Geometry check sheet. Reference: the model listing, model coordinates, mm. Face numbers are marked on the shaded views. A direction names the side the tool comes from. Coordinates: 2 decimals unless noted, no trailing zeros. Order: outer loops, then holes, each group sorted by start corner. A loop starts at its lowest first (then second) coordinate and runs counter-clockwise, first axis right, second up. Notation, with made-up numbers: M 76.5,-20.75 L 89.5,-20.75 A8 cw 89.5,-15.75 Z; hole C 58,69.25 d8. An arc over 180 degrees is marked long. One line per item, written item: value. Start each with the question number.
1) Access from +Z, -Z, +X, -X, +Y, -Y to the whole of each face (thin tool, end or side, straight path). Record for the marked faces 1 and 2.
2) Sectioned sample at B-B, the plane x = 0. Enter the section's corners in (y, z).
3) Go/stop test with a flat-tipped pin: P1, Ø9, axis at x = 0, y = 0, coming from the +Z side (3 decimals). Record where the tip stops, or that it passes through.
4) Thickness scan on L1, parallel to Y at x = 0, z = 15; L2, parallel to X at y = 0, z = 1.15; L3, parallel to Y at x = 0, z = 1.35. Record the ranges inside material, lowest first. Write a range as from..to.
5) Sectioned sample at D-D, the plane z = 10.75. Enter the section's corners in (x, y), then the cut area to 3 significant figures.
6) Sectioned sample at C-C, the plane x = 15. Enter the section's corners in (y, z), then the cut area to 3 significant figures.
7) Sectioned sample at A-A, the plane y = -1.75. Enter the section's corners in (x, z), then the cut area to 3 significant figures.
8) Draft check along Y on the marked faces 3, 4, 5 and 6. Enter one of: pulls with the +Y half, pulls with the -Y half, needs draft (parallel to the pull), parting line crosses it, or undercut.
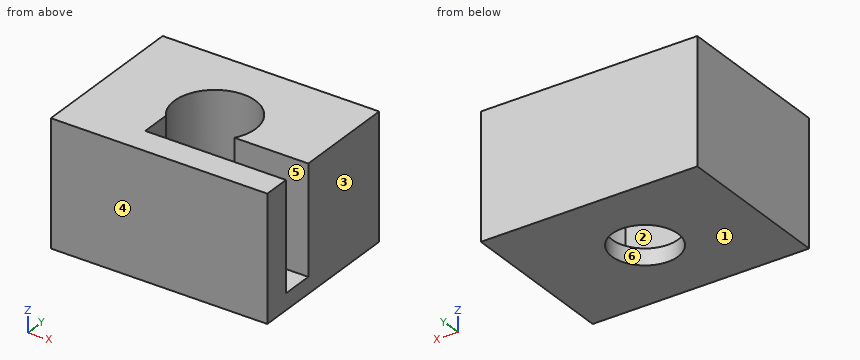
```python
from build123d import *

# Parameters (mm, degrees)
SKETCH1_W           = 40
SKETCH1_H           = 30
BOSS_EXTRUDE1_DEPTH = 23
SKETCH3_R           = 6.1
CUT_EXTRUDE1_DEPTH  = 24
CUT_EXTRUDE2_DEPTH  = 20


with BuildPart() as part:
    # Sketch1 → Boss-Extrude1 (new body)
    with BuildSketch(Plane.XY):
        Rectangle(SKETCH1_W, SKETCH1_H)
    extrude(amount=BOSS_EXTRUDE1_DEPTH)

    # Sketch3 → Cut-Extrude1 (cut, through all)
    with BuildSketch(Plane.XY.offset(23)):
        Circle(SKETCH3_R)
    extrude(amount=-CUT_EXTRUDE1_DEPTH, mode=Mode.SUBTRACT)

    # Sketch4 → Cut-Extrude2 (cut)
    with BuildSketch(Plane.XY.offset(23)):
        with BuildLine():
            Line((-6, -4.5), (-6, -4))
            Line((-6, -4), (-4.605431576, -4))
            ThreePointArc((-4.605431576, -4), (-2.135048874, 5.714154907), (6.1, 0))
            ThreePointArc((6.1, 0), (5.714154907, -2.135048874), (4.605431576, -4))
            Line((4.605431576, -4), (6.34428877, -4))
            ThreePointArc((6.34428877, -4), (7.205281597, -2.081806214), (7.5, 0))
            ThreePointArc((7.5, 0), (-2.371708245, 7.115124735), (-6, -4.5))
        make_face()
        with BuildLine():
            Line((-4.605431576, -4), (-6, -4))
            Line((-6, -4), (-6, -4.5))
            ThreePointArc((-6, -4.5), (0.303535318, -7.493855237), (6.34428877, -4))
            Line((6.34428877, -4), (4.605431576, -4))
            ThreePointArc((4.605431576, -4), (0, -6.1), (-4.605431576, -4))
        make_face()
        with BuildLine():
            ThreePointArc((6.34428877, -4), (0.303535318, -7.493855237), (-6, -4.5))
            Line((-6, -4.5), (-6, -10))
            Line((-6, -10), (20, -10))
            Line((20, -10), (20, -4))
            Line((20, -4), (6.34428877, -4))
        make_face()
    extrude(amount=-CUT_EXTRUDE2_DEPTH, mode=Mode.SUBTRACT)


solid = part.part
```
Final values:
1. face 1: -Z, +X, -X, +Y, -Y
1. face 2: +Z, +X
2. outline: M -15,0 L -6.1,0 L -6.1,3 L -10,3 L -10,23 L -15,23 Z; M 6.1,0 L 15,0 L 15,23 L 7.5,23 L 7.5,3 L 6.1,3 Z
3. P1: passes through
4. L1: y = -15..-10, 7.5..15
4. L2: x = -20..-6.1, 6.1..20
4. L3: y = -15..-6.1, 6.1..15
5. outline: M -20,-15 L 20,-15 L 20,-10 L -6,-10 L -6,-4.5 A7.5 cw long 6.34,-4 L 20,-4 L 20,15 L -20,15 Z
5. area: 899 mm^2
6. outline: M -15,0 L 15,0 L 15,23 L -4,23 L -4,3 L -10,3 L -10,23 L -15,23 Z
6. area: 570 mm^2
7. outline: M -20,0 L -5.84,0 L -5.84,3 L -7.29,3 L -7.29,23 L -20,23 Z; M 5.84,0 L 20,0 L 20,23 L 7.29,23 L 7.29,3 L 5.84,3 Z
7. area: 593 mm^2
8. face 3: needs draft
8. face 4: pulls with the -Y half
8. face 5: undercut
8. face 6: undercut
